Check sheet for the modelled part. Datum: model origin and axes. Units: mm. Give positions to 0.01 mm unless a question says otherwise; leave off trailing zeros. Order: outer loops, then holes, each group sorted by start corner. A loop starts at its lowest first (then second) coordinate and runs counter-clockwise, first axis right, second up. Notation, with made-up numbers: (15.25, -11.5) -> (34.25, -11.5) arc R26 cw to (34.25, 14.5) -> close; hole circle Ø7 at (68, 81). An arc over 180 degrees is marked (long way). Write each question's results on one line, items separated by ' | '.
from build123d import *

# Parameters (mm, degrees)
SKETCH_1_R          = 3.75
SKETCH_1_R_2        = 1.6
EXTRUDE_1_DEPTH     = 7
SKETCH_2_W          = 7
SKETCH_2_H          = 0.15
EXTRUDE_2_DEPTH     = 50
SKETCH_3_R          = 1.6
CUT_EXTRUDE_1_DEPTH = 52.019824578


with BuildPart() as part:
    # 草图1 → 凸台-拉伸1 (new body)
    with BuildSketch(Plane(origin=(0, 0, 0), x_dir=(0, 0, -1), z_dir=(1, 0, 0))):
        Circle(SKETCH_1_R)
        Circle(SKETCH_1_R_2, mode=Mode.SUBTRACT)
    extrude(amount=EXTRUDE_1_DEPTH)

    # 草图2 → 凸台-拉伸2 (add)
    with BuildSketch(Plane(origin=(0, 0, 0), x_dir=(1, 0, 0), z_dir=(0, 1, 0))):
        with Locations((3.5, 3.675)):
            Rectangle(SKETCH_2_W, SKETCH_2_H)
    extrude(amount=-EXTRUDE_2_DEPTH)

    # 草图3 → 切除-拉伸1 (cut, through all)
    with BuildSketch(Plane.XY.offset(-3.6)):
        with Locations((3.5, -46.8)):
            Circle(SKETCH_3_R)
    extrude(amount=-CUT_EXTRUDE_1_DEPTH, mode=Mode.SUBTRACT)


solid = part.part
1. Material ranges on probe 1 along Y at (x, z) = (3.25, 0); probe 2 along Y at (x, z) = (5.75, -2.75); probe 3 along Y at (x, z) = (3.5, 3.25), recorded low to high. Write a range as from..to.
Verdict:
probe 1: y = -3.75..-1.6, 1.6..3.75 | probe 2: y = -2.55..2.55 | probe 3: y = -1.87..1.87
2. Mould release check, pull along Y, two halves, no side actions. Record for faces 1 (the flat face through (3, -25, -3.75)), 2 (the cylindrical face through (3.45, -0.97, 1.27)): +Y half, -Y half, draft (parallel to the pull), parting line (faces both ways), or undercut.
Verdict:
face 1: draft | face 2: undercut
3. Gauge pin test, flat end, axial feed: pin 1 Ø1.5 at (x, z) = (3, -0.5) entering from -Y. Record the tip position at first contact, or that the pin passes through.
Verdict:
pin 1: stops at y = -3.75
4. Section check D-D on x = 5.75. Record the cut outline in (y, z), then the cut area to 3 significant figures.
Verdict:
outline: (-50, -3.75) -> (0, -3.75) arc R3.75 ccw (long way) to (-1.05, -3.6) -> (-50, -3.6) -> close; hole circle Ø3.2 at (0, 0) | area: 43.5 mm^2
5. Section check A-A on x = 3.5. Record the cut outline in (y, z).
Verdict:
outline: (-50, -3.75) -> (-48.4, -3.75) -> (-48.4, -3.6) -> (-50, -3.6) -> close; (-45.2, -3.75) -> (0, -3.75) arc R3.75 ccw (long way) to (-1.05, -3.6) -> (-45.2, -3.6) -> close; hole circle Ø3.2 at (0, 0)
6. Section check B-B on y = -46.8. Record the cut outline in (x, z).
Verdict:
outline: (0, -3.75) -> (1.9, -3.75) -> (1.9, -3.6) -> (0, -3.6) -> close; (5.1, -3.75) -> (7, -3.75) -> (7, -3.6) -> (5.1, -3.6) -> close
7. Section check C-C on z = 0. Record the cut outline in (x, y), then the cut area to 3 significant figures.
Verdict:
outline: (0, -3.75) -> (7, -3.75) -> (7, -1.6) -> (0, -1.6) -> close; (0, 1.6) -> (7, 1.6) -> (7, 3.75) -> (0, 3.75) -> close | area: 30.1 mm^2
